```python
from build123d import *

# Parameters (mm, degrees)
F0_R      = 50.8
F1_DEPTH  = 6.35
F2_R      = 6.223
F3_DEPTH  = 50.8
F4_W      = 152.4
F4_H      = 76.2
F5_DEPTH  = 6.35
F6_R      = 1.5875
F7_DEPTH  = 6.35
F8_R      = 1.5875
F9_DEPTH  = 6.35
F10_R     = 1.5875
F11_DEPTH = 25.4


with BuildPart() as f1:
    # F0 (on Top) → F1 (new body)
    with BuildSketch(Plane.XY):
        Circle(F0_R)
    extrude(amount=F1_DEPTH)

    # F2 (on face) → F3 (join)
    with BuildSketch(Plane.XY.offset(6.35)):
        with Locations((0, -36.5125)):
            Circle(F2_R)
        with Locations((0, 36.5125)):
            Circle(F2_R)
    extrude(amount=F3_DEPTH)

    # F4 (on Top) → F5 (join)
    with BuildSketch(Plane.XY):
        Rectangle(F4_W, F4_H)
    extrude(amount=F5_DEPTH)

    # F6 (on face) → F7 (cut, through all)
    with BuildSketch(Plane.XY.offset(6.35)):
        with Locations((-53.975, 26.9875)):
            Circle(F6_R)
        with Locations((-69.85, -23.01875)):
            Circle(F6_R)
        with Locations((-26.19375, 26.9875)):
            Circle(F6_R)
        with Locations((-21.43125, -24.60625)):
            Circle(F6_R)
        with Locations((25.4, 22.225)):
            Circle(F6_R)
        with Locations((69.85, 22.225)):
            Circle(F6_R)
        with Locations((25.4, -22.225)):
            Circle(F6_R)
        with Locations((69.85, -22.225)):
            Circle(F6_R)
    extrude(amount=-F7_DEPTH, mode=Mode.SUBTRACT)

    # F8 (on face) → F9 (cut)
    with BuildSketch(Plane.XY.offset(57.15)):
        with Locations((0, 36.5125)):
            Circle(F8_R)
        with Locations((0, -36.5125)):
            Circle(F8_R)
    extrude(amount=-F9_DEPTH, mode=Mode.SUBTRACT)

    # F10 (on face) → F11 (cut)
    with BuildSketch(Plane.XY.offset(6.35)):
        with Locations((-69.85, 31.75)):
            Circle(F10_R)
        with Locations((-69.85, -31.75)):
            Circle(F10_R)
        with Locations((69.85, -31.75)):
            Circle(F10_R)
        with Locations((69.85, 31.75)):
            Circle(F10_R)
    extrude(amount=-F11_DEPTH, mode=Mode.SUBTRACT)


solid = f1.part
```
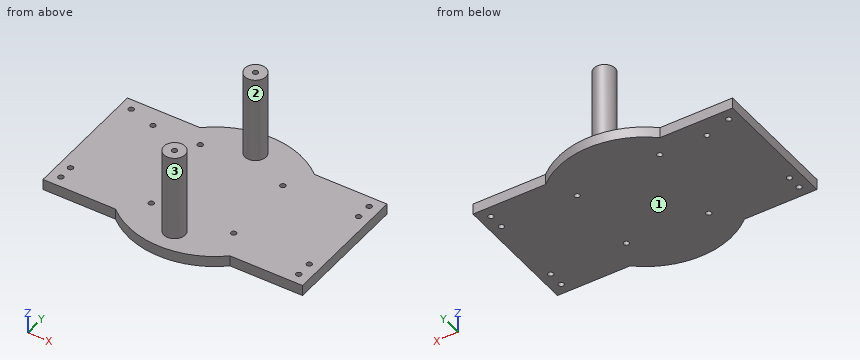
Build history of the part. All positions in model axes, mm. Face numbers are marked on the shaded views. Give positions to 0.01 mm unless a question says otherwise; leave off trailing zeros. Order: outer loops, then holes, each group sorted by start corner. A loop starts at its lowest first (then second) coordinate and runs counter-clockwise, first axis right, second up. Notation, with made-up numbers: M 50.25,46.25 L 85.25,46.25 A16 cw 85.25,62.25 Z; hole C 13.5,64 d3. An arc over 180 degrees is marked long. Write item = value, one per line. Start each with the question number.
(1) Slice it at A-A on x = -69.85. Write the cut outline in (y, z), plus the area to 3 significant figures.
(2) Probe L1, parallel to Y at x = 69.85, z = 2.25; L2, parallel to X at y = -31, z = 1; L3, parallel to Y at x = 69, z = 3. List the from-to ranges inside material, lowest first. Write a range as [from, to].
(3) Slice it at D-D on z = 52.5. Write the cut outline in (x, y) (1 decimal).
(4) Two-plate mould, pull along Y, no slides. Class the marked faces 1, 2 and 3: released by +Y, released by -Y, zero draft, split by the parting line, or undercut.
(5) Slice it at B-B on x = 69.85. Write the cut outline in (y, z).
(6) Pin check, flat tips, straight feed: pin 1 Ø8 at (y, z) = (-38, 41.5) entering from +X; pin 2 Ø3 at (x, y) = (25.4, 22.225) entering from +Z; pin 3 Ø4 at (x, y) = (-53.98, 26.99) entering from +Z; pin 4 Ø7 at (x, z) = (-46, 4) entering from +Y. Stop position of each tip, or through.
Responses:
q1.outline = M -38.1,0 L -33.34,0 L -33.34,6.35 L -38.1,6.35 Z; M -30.16,0 L -24.61,0 L -24.61,6.35 L -30.16,6.35 Z; M -21.43,0 L 30.16,0 L 30.16,6.35 L -21.43,6.35 Z; M 33.34,0 L 38.1,0 L 38.1,6.35 L 33.34,6.35 Z
q1.area = 423 mm2
q2.L1 = [-38.1, -33.34], [-30.16, -23.81], [-20.64, 20.64], [23.81, 30.16], [33.34, 38.1]
q2.L2 = [-76.2, -71.25], [-68.45, 68.45], [71.25, 76.2]
q2.L3 = [-38.1, -33.09], [-30.41, -23.57], [-20.88, 20.88], [23.57, 30.41], [33.09, 38.1]
q3.outline = C 0,-36.5 d12.4; C 0,36.5 d12.4; hole C 0,-36.5 d3.2; hole C 0,36.5 d3.2
q4.face_1 = zero draft
q4.face_2 = undercut
q4.face_3 = undercut
q5.outline = M -38.1,0 L -33.34,0 L -33.34,6.35 L -38.1,6.35 Z; M -30.16,0 L -23.81,0 L -23.81,6.35 L -30.16,6.35 Z; M -20.64,0 L 20.64,0 L 20.64,6.35 L -20.64,6.35 Z; M 23.81,0 L 30.16,0 L 30.16,6.35 L 23.81,6.35 Z; M 33.34,0 L 38.1,0 L 38.1,6.35 L 33.34,6.35 Z
q6.pin_1 = 6.22
q6.pin_2 = through
q6.pin_3 = 6.35
q6.pin_4 = 38.1
